Verification items for the finished model (mm, model axes). Face numbers are marked on the shaded views. A direction names the side the tool comes from. Give positions to 0.01 mm unless a question says otherwise; leave off trailing zeros. Write each loop counter-clockwise with the first axis right and the second up, starting at its lowest first coordinate (ties: lowest second). Pieces come first, ordered by that corner, then holes. Notation, with made-up numbers: (76.25, 57.5) -> (132.25, 57.5) arc R11 cw to (132.25, 76.5) -> close; hole circle Ø3 at (9, 85). An arc over 180 degrees is marked (long way). Write item = value, one per line.
from build123d import *

# Parameters (mm, degrees)
F0_W     = 15
F0_H     = 18.1881040335
F0_W_2   = 20.5
F1_DEPTH = 7
F3_SIZE2 = 2
F3_SIZE  = 10
F4_R     = 5
F5_R     = 9.1937545257
F6_DEPTH = 7
F7_R     = 5


with BuildPart() as f1:
    # F0 (on Front) → F1 (new body)
    with BuildSketch(Plane.XZ):
        with BuildLine():
            Line((-20.5, 0), (0, 0))
            Line((0, 0), (0, 22.5676391274))
            Line((0, 22.5676391274), (-49.5, 22.5676391274))
            Line((-49.5, 22.5676391274), (-49.5, 0))
            Line((-49.5, 0), (-34.5, 0))
            ThreePointArc((-34.5, 0), (-27.5, 7), (-20.5, 0))
        make_face()
        with Locations((-42, -9.0940520167)):
            Rectangle(F0_W, F0_H)
        with Locations((-10.25, -9.0940520167)):
            Rectangle(F0_W_2, F0_H)
        with BuildLine():
            Line((0, 22.5676391274), (0, 0))
            Line((0, 0), (20.5, 0))
            ThreePointArc((20.5, 0), (27.5, 7), (34.5, 0))
            Line((34.5, 0), (49.5, 0))
            Line((49.5, 0), (49.5, 22.5676391274))
            Line((49.5, 22.5676391274), (0, 22.5676391274))
        make_face()
        with Locations((10.25, -9.0940520167)):
            Rectangle(F0_W_2, F0_H)
        with Locations((42, -9.0940520167)):
            Rectangle(F0_W, F0_H)
    extrude(amount=F1_DEPTH)

    # F3
    f3_edges = [f1.edges().sort_by_distance(p)[0] for p in [
        (0, 0, -18.188104),
        (42, 0, -18.188104),
        (-42, 0, -18.188104),
    ]]
    f3_side = f1.faces().sort_by_distance((0, 0, 3.858473))[0]
    chamfer(f3_edges, length=F3_SIZE, length2=F3_SIZE2, reference=f3_side)

    # F4
    f4_edges = [f1.edges().sort_by_distance(p)[0] for p in [
        (-20.5, -4.5, -18.188104),
        (-34.5, -4.5, -18.188104),
        (20.5, -4.5, -18.188104),
        (34.5, -4.5, -18.188104),
        (49.5, -4.5, -18.188104),
        (-49.5, -4.5, -18.188104),
    ]]
    fillet(f4_edges, radius=F4_R)

    # F5 (on Front) → F6 (cut, through all)
    with BuildSketch(Plane.XZ):
        with Locations((-27.5, 0)):
            Circle(F5_R)
        with Locations((27.5, 0)):
            Circle(F5_R)
    extrude(amount=F6_DEPTH, mode=Mode.SUBTRACT)

    # F7
    f7_edges = [f1.edges().sort_by_distance(p)[0] for p in [
        (-49.5, -3.5, 22.567639),
        (49.5, -3.5, 22.567639),
    ]]
    fillet(f7_edges, radius=F7_R)


solid = f1.part
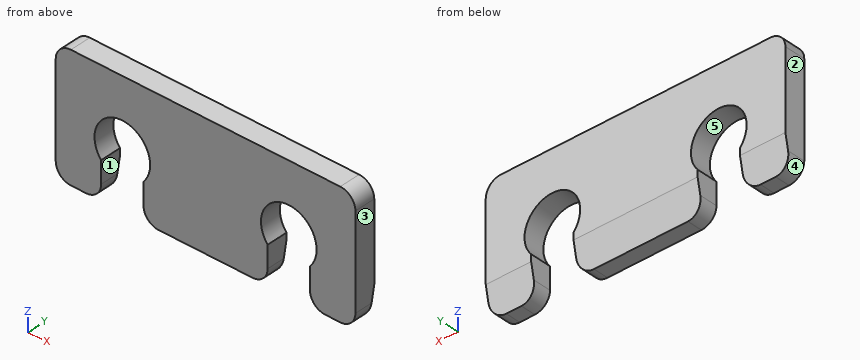
Item 1: Material ranges on line 1 (X direction, y = -3.25, z = 0); line 2 (X direction, y = -4.5, z = -11); line 3 (Z direction, x = -27.5, y = -5.5), recorded low to high.
Response values:
line_1 = -49.5 to -36.69, -18.31 to 18.31, 36.69 to 49.5
line_2 = -49.5 to -34.5, -20.5 to 20.5, 34.5 to 49.5
line_3 = 9.19 to 22.57
Item 2: Sectioned sample at C-C on x = -27.5. Record the cut outline in (y, z).
Response values:
outline = (-7, 9.19) -> (0, 9.19) -> (0, 22.57) -> (-7, 22.57) -> close
Item 3: Mould release check, pull along Z, two halves, no side actions. Record for the marked faces 3, 4 and 5: +Z half, -Z half, draft (parallel to the pull), parting line (faces both ways), or undercut.
Response values:
face_3 = draft
face_4 = -Z half
face_5 = undercut
Item 4: Sectioned sample at D-D on z = -11.5. Record the cut outline in (x, y), then the cut area to 3 significant figures.
Response values:
outline = (-49.5, -7) -> (-34.5, -7) -> (-34.5, -0.66) -> (-49.5, -0.66) -> close; (-20.5, -7) -> (20.5, -7) -> (20.5, -0.66) -> (-20.5, -0.66) -> close; (34.5, -7) -> (49.5, -7) -> (49.5, -0.66) -> (34.5, -0.66) -> close
area = 450 mm^2
Item 5: Go/stop test with a flat-tipped pin: P1, Ø10, axis at x = 35.5, z = 0, coming from the -Y side. Record where the tip stops, or that it passes through.
Response values:
P1 = -7
Item 6: Set-up check for the marked faces 1 and 2: record each of +Z, -Z, +X, -X, +Y, -Y from which the full face is reachable in a straight line by a thin tool's end or side.
Response values:
face_1 = -Z, +Y, -Y
face_2 = +Z, -Z, -X, +Y, -Y
Item 7: Sectioned sample at B-B on y = -4.75. Record the cut outline in (x, z), then the cut area to 3 significant figures.
Response values:
outline = (-49.5, -13.19) arc R5 ccw to (-44.5, -18.19) -> (-39.5, -18.19) arc R5 ccw to (-34.5, -13.19) -> (-34.5, -5.96) arc R9.19 cw (long way) to (-20.5, -5.96) -> (-20.5, -13.19) arc R5 ccw to (-15.5, -18.19) -> (15.5, -18.19) arc R5 ccw to (20.5, -13.19) -> (20.5, -5.96) arc R9.19 cw (long way) to (34.5, -5.96) -> (34.5, -13.19) arc R5 ccw to (39.5, -18.19) -> (44.5, -18.19) arc R5 ccw to (49.5, -13.19) -> (49.5, 17.57) arc R5 ccw to (44.5, 22.57) -> (-44.5, 22.57) arc R5 ccw to (-49.5, 17.57) -> close
area = 3,180 mm^2
Item 8: Sectioned sample at A-A on z = 0. Record the cut outline in (x, y), then the cut area to 3 significant figures.
Response values:
outline = (-49.5, -7) -> (-36.69, -7) -> (-36.69, 0) -> (-49.5, 0) -> close; (-18.31, -7) -> (18.31, -7) -> (18.31, 0) -> (-18.31, 0) -> close; (36.69, -7) -> (49.5, -7) -> (49.5, 0) -> (36.69, 0) -> close
area = 436 mm^2
